Geometry: see drawing. Coordinates: mm, zero at the bounding-box minimum. A direction names the side the tool comes from. Give positions to 0.01 mm unless a question says otherwise; leave off trailing zeros. Write each loop counter-clockwise with the first axis right and the second up, starting at its lowest first coordinate (ties: lowest second). Pieces come first, ordered by that corner, then holes. Notation, with made-up numbers: (-16, 11.5) - (-10, 11.5) arc R24 ccw to (-10, 48.5) - close; hole circle Ø5 at (13, -30). An arc over 180 degrees is marked (long way). Return JSON: item names as keys, results as strings.
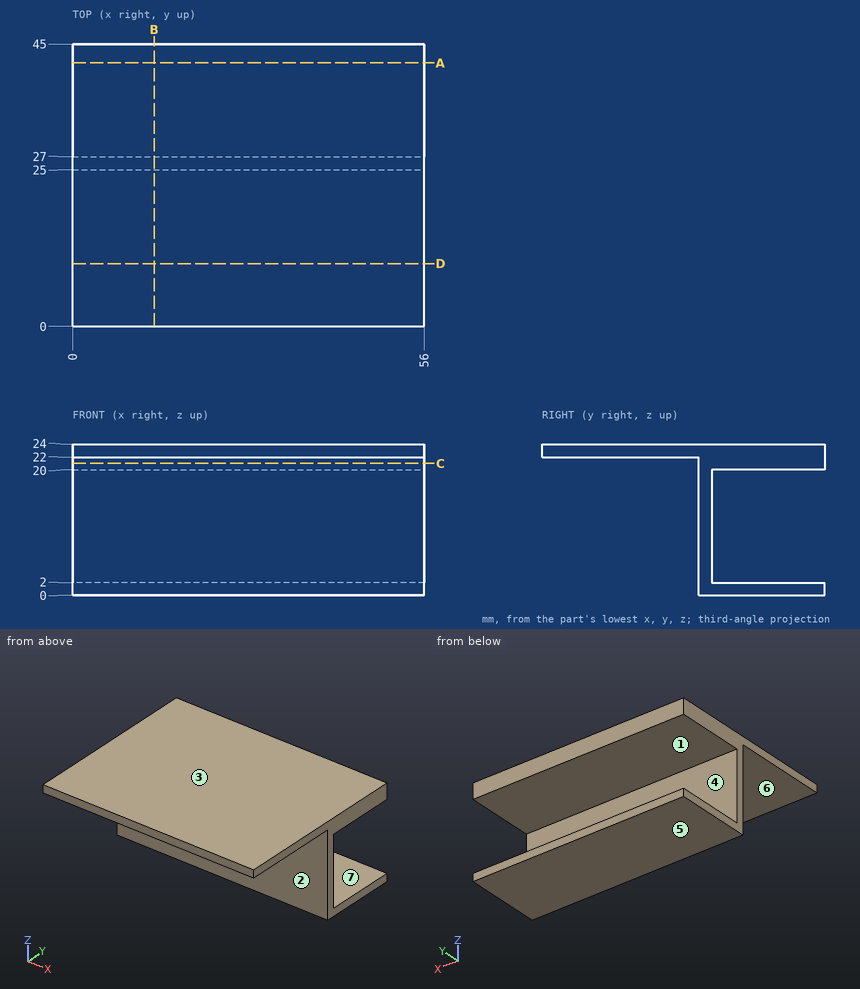
Q1. Set-up query: the marked faces 5, 6 and 7. Return all of +Z, -Z, +X, -X, +Y, -Y with unobstructed straight access to the full face (end or side cutting, diameter ignored); none if empty.
Answer key:
{"face 5": "-Z, +X, -X, +Y, -Y", "face 6": "-Z, +X, -X, -Y", "face 7": "+X, -X, +Y"}
Q2. Section query B-B, the plane x = 13. Return the cut outline in (y, z), plus the area to 3 significant figures.
Answer key:
{"outline": "(0, 22) - (25, 22) - (25, 0) - (45, 0) - (45, 2) - (27, 2) - (27, 20) - (45, 20) - (45, 24) - (0, 24) - close", "area": "206 mm^2"}
Q3. Mould query, pull axis Z, two halves, no side actions, for the marked faces 1, 2, 3 and 4. Classes: pulls with the +Z half, pulls with the -Z half, needs draft (parallel to the pull), parting line crosses it, or undercut.
Answer key:
{"face 1": "undercut", "face 2": "needs draft", "face 3": "pulls with the +Z half", "face 4": "undercut"}
Q4. Pin query (flat end, axial travel): P1, Ø5, axis at x = 12, z = 10, coming from the +Y side; P2, Ø7.5, axis at x = 38, y = 17.5, coming from the -Z side; P3, Ø2, axis at x = 29, z = 17, coming from the -Y side. Return the tip coordinate at first contact, or that it passes through.
Answer key:
{"P1": "stops at y = 27", "P2": "stops at z = 22", "P3": "stops at y = 25"}
Q5. Section query C-C, the plane z = 21. Return the cut outline in (x, y), plus the area to 3 significant figures.
Answer key:
{"outline": "(0, 25) - (56, 25) - (56, 45) - (0, 45) - close", "area": "1,120 mm^2"}
Q6. Material intervals for probe 1 along Z at (x, y) = (32, 35); probe 2 along Z at (x, y) = (21.5, 8); probe 3 along Y at (x, z) = (5, 5.75), sorted ascending. Write a range as [from, to].
Answer key:
{"probe 1": "z = [0, 2], [20, 24]", "probe 2": "z = [22, 24]", "probe 3": "y = [25, 27]"}
Q7. Section query A-A, the plane y = 42. Return the cut outline in (x, z).
Answer key:
{"outline": "(0, 0) - (56, 0) - (56, 2) - (0, 2) - close; (0, 20) - (56, 20) - (56, 24) - (0, 24) - close"}
Q8. Section query D-D, the plane y = 10. Return the cut outline in (x, z).
Answer key:
{"outline": "(0, 22) - (56, 22) - (56, 24) - (0, 24) - close"}
